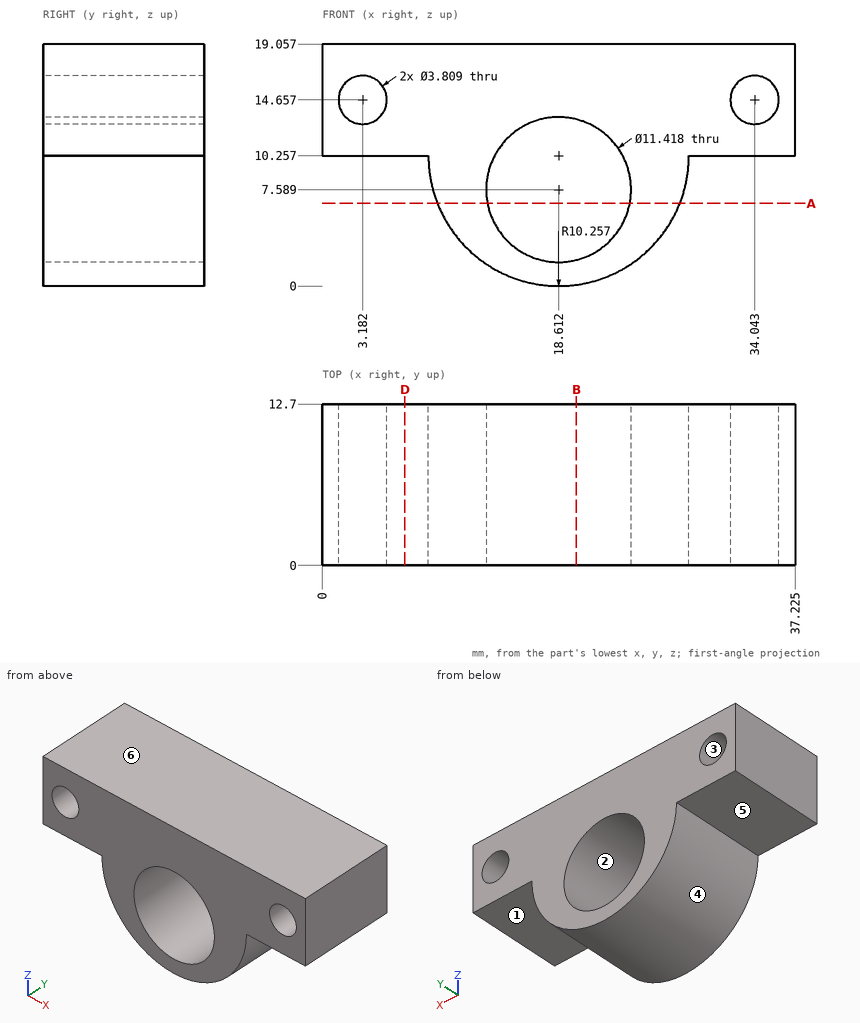
Answer from the drawing. Dimensions are ordinates in mm from the lowest x, y and z of the part. A direction names the side the tool comes from. Coordinates: 2 decimals unless noted, no trailing zeros. Loops run counter-clockwise (first coordinate to the right, second up) from the corner with the lowest first, then second, coordinate; pieces in that order, holes last. Notation, with made-up numbers: (10, -33.5) -> (58, -33.5) arc R5 cw to (58, -27.5) -> close; hole circle Ø4 at (57.5, 48). An arc over 180 degrees is marked (long way). Return JSON: item names as keys, results as strings.
Item 1: For the marked faces 5 and 6, determine the directions among +Z, -Z, +X, -X, +Y, -Y from which every point of the face is accessible in a straight line to the end or side of a thin tool.
Answers:
{"face 5": "-Z, -X, +Y, -Y", "face 6": "+Z, +X, -X, +Y, -Y"}
Item 2: Find the intervals of material crossed by probe 1 along X at (y, z) = (11, 14.5) (1 decimal); probe 2 along X at (y, z) = (6.75, 16) (1 decimal); probe 3 along Z at (x, y) = (7.5, 1), in increasing order.
Answers:
{"probe 1": "x = 0 to 1.3, 5.1 to 32.1, 35.9 to 37.2", "probe 2": "x = 0 to 1.8, 4.5 to 32.7, 35.4 to 37.2", "probe 3": "z = 10.26 to 19.06"}
Item 3: For a pull along X with two mould halves and no side action, classify the marked faces 1, 2, 3 and 4 as +X half, -X half, draft (parallel to the pull), parting line (faces both ways), or undercut.
Answers:
{"face 1": "draft", "face 2": "undercut", "face 3": "undercut", "face 4": "parting line"}
Item 4: Find section B-B (x = 20). Determine the outline of the cut face in (y, z) (1 decimal).
Answers:
{"outline": "(0, 0.1) -> (12.7, 0.1) -> (12.7, 2.1) -> (0, 2.1) -> close; (0, 13.1) -> (12.7, 13.1) -> (12.7, 19.1) -> (0, 19.1) -> close"}
Item 5: Find section A-A (z = 6.5). Determine the outline of the cut face in (x, y).
Answers:
{"outline": "(9.07, 0) -> (13.01, 0) -> (13.01, 12.7) -> (9.07, 12.7) -> close; (24.22, 0) -> (28.16, 0) -> (28.16, 12.7) -> (24.22, 12.7) -> close"}
Item 6: Flat-ended cylindrical pins translate along their axes: P1, Ø6, axis at x = 25.5, y = 2, coming from the -Z side (1 decimal); P2, Ø6.5, axis at x = 35, y = 6.5, coming from the -Z side; P3, Ø4, axis at y = 10, z = 6.5, coming from the -X side; P4, Ø6, axis at x = 34.04, z = 14.66, coming from the +Y side. Find the tip coordinate at first contact, or state that the pin passes through.
Answers:
{"P1": "stops at z = 0.8", "P2": "stops at z = 10.26", "P3": "stops at x = 8.51", "P4": "stops at y = 12.7"}
Item 7: Find section D-D (x = 6.5). Determine the outline of the cut face in (y, z).
Answers:
{"outline": "(0, 10.26) -> (12.7, 10.26) -> (12.7, 19.06) -> (0, 19.06) -> close"}
